```python
from build123d import *

# Parameters (mm, degrees)
SKETCH1_W                   = 15
SKETCH1_H                   = 15
BOSS_EXTRUDE1_DEPTH         = 40
CUT_EXTRUDE1_DEPTH          = 44.373378932
SKETCH3_W                   = 25
SKETCH3_H                   = 25
BOSS_EXTRUDE2_DEPTH         = 300
F_1_4_0_25_DIAMETER_HOLE1_D = 6.35


with BuildPart() as part:
    # Sketch1 → Boss-Extrude1 (new body)
    with BuildSketch(Plane(origin=(0, 0, 0), x_dir=(1, 0, 0), z_dir=(0, 1, 0))):
        Rectangle(SKETCH1_W, SKETCH1_H)
    extrude(amount=BOSS_EXTRUDE1_DEPTH)

    # Sketch2 → Cut-Extrude1 (cut, through all)
    with BuildSketch(Plane.XY.offset(7.5)):
        with BuildLine():
            ThreePointArc((1.6e-07, 0), (-3.820345171, 0.368266435), (-7.5, 1.459503782))
            Line((-7.5, 1.459503782), (-7.5, 0))
            Line((-7.5, 0), (1.6e-07, 0))
        make_face()
        with BuildLine():
            ThreePointArc((7.5, 1.459503782), (3.820345328, 0.368266465), (1.6e-07, 0))
            Line((1.6e-07, 0), (7.5, 0))
            Line((7.5, 0), (7.5, 1.459503782))
        make_face()
    extrude(amount=-CUT_EXTRUDE1_DEPTH, mode=Mode.SUBTRACT)

    # Sketch3 → Boss-Extrude2 (add)
    with BuildSketch(Plane(origin=(0, 40, 0), x_dir=(1, 0, 0), z_dir=(0, 1, 0))):
        Rectangle(SKETCH3_W, SKETCH3_H)
    extrude(amount=BOSS_EXTRUDE2_DEPTH)

    # 1/4 (0.25) Diameter Hole1 (through all)
    with Locations(Plane(origin=(12.5, 0, 0), x_dir=(0, 0, -1), z_dir=(1, 0, 0))):
        with Locations((0, 325)):
            Hole(F_1_4_0_25_DIAMETER_HOLE1_D / 2)


solid = part.part
```
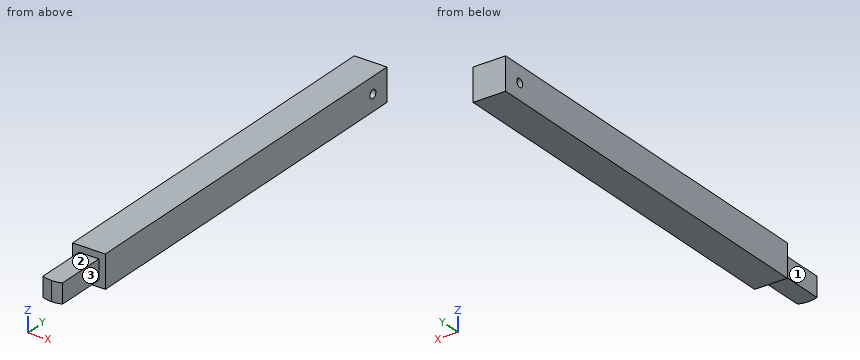
Part model, mm, in its own coordinate system. Face numbers are marked on the shaded views. A direction names the side the tool comes from. Round coordinates to 2 decimals unless told otherwise and drop trailing zeros. Loops run counter-clockwise (first coordinate to the right, second up) from the corner with the lowest first, then second, coordinate; pieces in that order, holes last.
Item 1: Drill centre lines: line 1 (Z direction, x = 5.75, y = 325) (3 decimals); line 2 (Y direction, x = 1.5, z = 0) (3 decimals); line 3 (Y direction, x = 8.5, z = -0.25). Where is each one in solid material? Low to high.
Item 2: Cut at B-B, the plane z = 0. Give the cut face in (x, y) (1 decimal).
Item 3: 3-axis set-ups, long thin cutter, end or side, ignore diameter. For the marked faces 1, 2 and 3: which of +Z, -Z, +X, -X, +Y, -Y reach the whole face in a straight line?
Item 4: Cut at A-A, the plane y = 325. Give the cut face in (x, z) (3 decimals).
Item 5: Drop flat-ended pins along their axis: P1, Ø6, axis at x = -8.5, z = 4, coming from the -Y side; P2, Ø5, axis at y = 325, z = 0, coming from the -X side; P3, Ø12, axis at y = 24.5, z = -2, coming from the +X side; P4, Ø12.5, axis at x = 2, z = -1, coming from the -Y side. Give the stop position or say it passes through.
A:
1. line 1: z = -12.5 to -3.175, 3.175 to 12.5
1. line 2: y = 0.056 to 321.825, 328.175 to 340
1. line 3: y = 40 to 321.83, 328.17 to 340
2. outline: (-12.5, 40) - (-7.5, 40) - (-7.5, 1.5) arc R20 ccw to (7.5, 1.5) - (7.5, 40) - (12.5, 40) - (12.5, 321.8) - (-12.5, 321.8) - close; (-12.5, 328.2) - (12.5, 328.2) - (12.5, 340) - (-12.5, 340) - close
3. face 1: +Z, -Z, -X, -Y
3. face 2: +Z, +X, -X, -Y
3. face 3: +Z, -Z, +X, -Y
4. outline: (-12.5, -12.5) - (12.5, -12.5) - (12.5, -3.175) - (-12.5, -3.175) - close; (-12.5, 3.175) - (12.5, 3.175) - (12.5, 12.5) - (-12.5, 12.5) - close
5. P1: stops at y = 0.77
5. P2: passes through
5. P3: stops at x = 7.5
5. P4: stops at y = 0
